from build123d import *

# Parameters (mm, degrees)
BOSS_EXTRUDE1_DEPTH = 17
BOSS_EXTRUDE2_DEPTH = 2
BOSS_EXTRUDE3_DEPTH = 2
SKETCH4_R           = 2.1
CUT_EXTRUDE1_DEPTH  = 100
CUT_EXTRUDE2_DEPTH  = 3
CUT_EXTRUDE3_DEPTH  = 6.5
CUT_EXTRUDE4_DEPTH  = 6.5
BOSS_EXTRUDE4_DEPTH = 4.5


with BuildPart() as part:
    # Sketch1 → Boss-Extrude1 (new body)
    with BuildSketch(Plane(origin=(0, 0, 0), x_dir=(1, 0, 0), z_dir=(0, 1, 0))):
        Polygon((-27.582659514, 44.185105583), (-2.582659514, 44.185105583), (-2.582659514, 38.185105583), (13.417340486, 38.185105583), (13.417340486, 42.685105583), (0.417340486, 42.685105583), (0.417340486, 54.185105583), (-30.582659514, 54.185105583), (-30.582659514, 42.685105583), (-43.582659514, 42.685105583), (-43.582659514, 38.185105583), (-27.582659514, 38.185105583), align=None)
    extrude(amount=BOSS_EXTRUDE1_DEPTH)

    # Sketch2 → Boss-Extrude2 (add)
    with BuildSketch(Plane(origin=(0, 17, 0), x_dir=(1, 0, 0), z_dir=(0, 1, 0))):
        Polygon((-43.582659514, 42.685105583), (-30.582659514, 54.185105583), (-30.582659514, 42.685105583), align=None)
        Polygon((0.417340486, 42.685105583), (13.417340486, 42.685105583), (0.417340486, 54.185105583), align=None)
    extrude(amount=-BOSS_EXTRUDE2_DEPTH)

    # Sketch3 → Boss-Extrude3 (add)
    with BuildSketch(Plane.XZ):
        Polygon((-43.582659514, -42.685105583), (-30.582659514, -54.185105583), (-30.582659514, -42.685105583), align=None)
        Polygon((0.417340486, -42.685105583), (0.417340486, -54.185105583), (13.417340486, -42.685105583), align=None)
    extrude(amount=-BOSS_EXTRUDE3_DEPTH)

    # Sketch4 → Cut-Extrude1 (cut)
    with BuildSketch(Plane.XY.offset(-38.185105583)):
        with Locations((-35.082659514, 8.5)):
            Circle(SKETCH4_R)
        with Locations((4.917340486, 8.5)):
            Circle(SKETCH4_R)
    extrude(amount=-CUT_EXTRUDE1_DEPTH, mode=Mode.SUBTRACT)

    # Sketch5 → Cut-Extrude2 (cut)
    with BuildSketch(Plane(origin=(0, 0, -42.685105583), x_dir=(-1, 0, 0), z_dir=(0, 0, -1))):
        Polygon((31.582659514, 6.479274058), (31.582659514, 10.520725942), (35.082659514, 12.541451884), (38.582659514, 10.520725942), (38.582659514, 6.479274058), (35.082659514, 4.458548116), align=None)
        Polygon((-1.417340486, 10.520725942), (-4.917340486, 12.541451884), (-8.417340486, 10.520725942), (-8.417340486, 6.479274058), (-4.917340486, 4.458548116), (-1.417340486, 6.479274058), align=None)
    extrude(amount=-CUT_EXTRUDE2_DEPTH, mode=Mode.SUBTRACT)

    # Sketch7 → Cut-Extrude3 (cut)
    with BuildSketch(Plane.ZY.offset(2.582659514)):
        with BuildLine():
            Line((-53.601964627, 19.27795803), (-35.36636136, 18.147314128))
            Line((-35.36636136, 18.147314128), (-35.36636136, -6.291096758))
            Line((-35.36636136, -6.291096758), (-39.347618514, -8.620327672))
            ThreePointArc((-39.347618514, -8.620327672), (-46.872397507, 5.125662458), (-53.601964627, 19.27795803))
        make_face()
    extrude(amount=CUT_EXTRUDE3_DEPTH, mode=Mode.SUBTRACT)

    # Sketch8 → Cut-Extrude4 (cut)
    with BuildSketch(Plane(origin=(-27.582659514, 0, 0), x_dir=(0, 0, -1), z_dir=(1, 0, 0))):
        with BuildLine():
            Line((60.133248532, 35.4590838), (29.94533861, 35.4590838))
            Line((29.94533861, 35.4590838), (34.196090785, -17.072827801))
            ThreePointArc((34.196090785, -17.072827801), (48.567589168, 8.50044914), (60.133248532, 35.4590838))
        make_face()
    extrude(amount=CUT_EXTRUDE4_DEPTH, mode=Mode.SUBTRACT)

    # Sketch9 → Boss-Extrude4 (add)
    with BuildSketch(Plane.XY.offset(-38.185105583)):
        with BuildLine():
            Line((-51.736745863, 12.379657112), (-54.233308347, 10.35))
            Line((-54.233308347, 10.35), (-56.336651381, 10.35))
            ThreePointArc((-56.336651381, 10.35), (-56.247164307, 11.045699168), (-55.569469191, 11.226626221))
            ThreePointArc((-55.569469191, 11.226626221), (-41.082659514, 8.5), (-55.569469191, 5.773373779))
            ThreePointArc((-55.569469191, 5.773373779), (-56.247164307, 5.954300832), (-56.336651381, 6.65))
            Line((-56.336651381, 6.65), (-54.233308347, 6.65))
            Line((-54.233308347, 6.65), (-51.736745863, 4.620342888))
            ThreePointArc((-51.736745863, 4.620342888), (-43.582659514, 8.5), (-51.736745863, 12.379657112))
        make_face()
    extrude(amount=-BOSS_EXTRUDE4_DEPTH)


solid = part.part
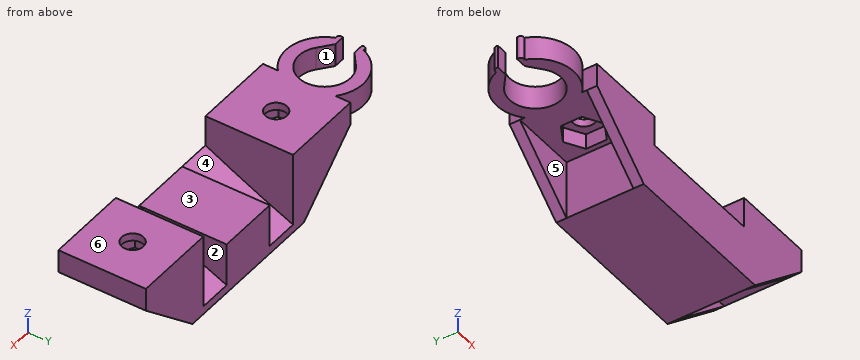
For this review, take the finished solid that the model builds, in its own axes (mm). Face numbers are marked on the shaded views. A direction names the side the tool comes from. Give positions to 0.01 mm unless a question says otherwise; leave off trailing zeros. Loops run counter-clockwise (first coordinate to the right, second up) from the corner with the lowest first, then second, coordinate; pieces in that order, holes last.
Item 1: Draft analysis for pull direction Y (two halves, no side actions). For the marked faces 4, 5 and 6, state which applies: +Y half, -Y half, draft (parallel to the pull), parting line (faces both ways), or undercut.
Item 2: For line 1 along X through (y, z) = (7, -46); line 2 along X through (y, z) = (8.5, -41.3); line 3 along Y through (x, z) = (-31, -47), list the stretches that pass through material, from the lowest coordinate up.
Item 3: Take a section at B-B, the plane x = -16. State the section outline as (y, z) points.
Item 4: Tool access review of the marked faces 1, 2 and 3: name each direction out of +Z, -Z, +X, -X, +Y, -Y from which nothing blocks a thin tool from reaching the whole face with its end or side.
Item 5: Take a section at A-A, the plane y = 7.5. Give the number of separate pieces and of enclosed holes in the cut face, and give its area (3 significant figures).
Item 6: Insertion check: pin 1 (8 mm diameter, centred on x = -38, z = -50.5, fed in from +Y); pin 2 (1 mm diameter, centred on y = 13, z = -46.5, fed in from -X); pin 3 (4 mm diameter, centred on y = 2, z = -52.5, fed in from +X); pin 4 (0.6 mm diameter, centred on x = -55.5, z = -40.5, fed in from -Y). Each pin has a flat end and moves straight along its axis. Give the tip position at first contact, or say it passes through.
Calculated:
1. face 4: +Y half
1. face 5: undercut
1. face 6: draft
2. line 1: x = -30.58 to -27.58, -21.08 to -9.08, -2.58 to 0.42
2. line 2: x = -43.58 to -38.58, -31.58 to -27.58, -2.58 to 1.42, 8.42 to 13.42
2. line 3: y = 0 to 2, 15 to 17
3. outline: (0, -54.19) - (17, -54.19) - (17, -44.19) - (0, -44.19) - close
4. face 1: +Z, -Z
4. face 2: +Z, +Y
4. face 3: +Z, +Y, -Y
5. separate pieces: 3
5. enclosed holes: 0
5. area: 360 mm2
6. pin 1: stops at y = 17
6. pin 2: stops at x = -30.58
6. pin 3: stops at x = 4.58
6. pin 4: stops at y = 4.97
